The drawing under review shows one solid part. Ordinate dimensions are in mm from its lowest x, y, z. A direction names the side the tool comes from. Coordinates: 2 decimals unless noted, no trailing zeros. Order: outer loops, then holes, each group sorted by start corner. A loop starts at its lowest first (then second) coordinate and runs counter-clockwise, first axis right, second up.
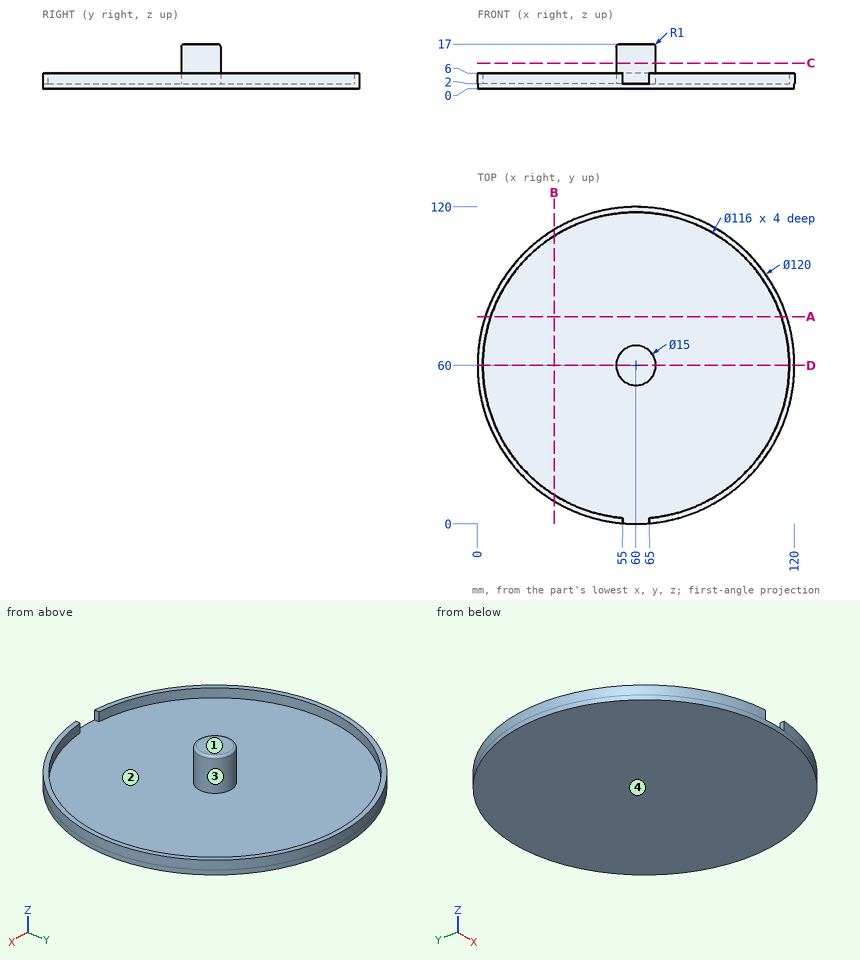
(1) Machinability: for the marked faces 3 and 4, which of the approach directions +Z, -Z, +X, -X, +Y, -Y give a long, thin tool a straight path to every point of the face, cutting with its end or side? Answer none if there is none.
A:
face 3: +Z
face 4: -Z, +X, -X, +Y, -Y
(2) For pin 1 Ø12 at (x, y) = (47.5, 25) entering from -Z; pin 2 Ø1.5 at (x, y) = (94, 90) entering from +Z; pin 3 Ø1.5 at (y, z) = (80.5, 3.5) entering from +X, all flat-tipped, find the tip position at first contact; note any pin that passes through.
A:
pin 1: stops at z = 0
pin 2: stops at z = 2
pin 3: stops at x = 116.66
(3) We need section C-C, the plane z = 9.75. Write out the cut boundary in (x, y), and give its area (3 significant figures).
A:
outline: circle Ø15 at (60, 60)
area: 177 mm2
(4) We need section A-A, the plane y = 78.5. Write out the cut boundary in (x, z).
A:
outline: (2.92, 0) - (117.08, 0) - (117.08, 6) - (114.97, 6) - (114.97, 2) - (5.03, 2) - (5.03, 6) - (2.92, 6) - close
(5) We need section B-B, the plane x = 29. Write out the cut boundary in (y, z).
A:
outline: (8.63, 0) - (111.37, 0) - (111.37, 6) - (109.02, 6) - (109.02, 2) - (10.98, 2) - (10.98, 6) - (8.63, 6) - close
(6) We need section D-D, the plane y = 60. Write out the cut boundary in (x, z).
A:
outline: (0, 0) - (120, 0) - (120, 6) - (118, 6) - (118, 2) - (67.5, 2) - (67.5, 16) arc R1 ccw to (66.5, 17) - (53.5, 17) arc R1 ccw to (52.5, 16) - (52.5, 2) - (2, 2) - (2, 6) - (0, 6) - close
(7) Wall thickness on probe 1 along Z at (x, y) = (36.5, 35.5); probe 2 along Y at (x, z) = (60, 16); probe 3 along X at (y, z) = (88, 3.25): over which ranges is each line inside the solid? List them lowest first.
A:
probe 1: z = 0 to 2
probe 2: y = 52.5 to 67.5
probe 3: x = 6.93 to 9.21, 110.79 to 113.07
(8) Draft analysis for pull direction X (two halves, no side actions). For the marked faces 1 and 2, state which applies: released by +X, released by -X, zero draft, split by the parting line, or undercut.
A:
face 1: zero draft
face 2: undercut
